Source: CAD feature listing. Evaluate the final solid. Frame: model axes, mm. A direction names the side the tool comes from. Coordinates: 2 decimals unless noted, no trailing zeros. Order: outer loops, then holes, each group sorted by start corner. A loop starts at its lowest first (then second) coordinate and runs counter-clockwise, first axis right, second up. Notation, with made-up numbers: (24.25, 28) - (73.25, 28) arc R31 ccw to (73.25, 62) - close; hole circle Ø3 at (66, 20.5). An arc over 180 degrees is marked (long way). One line per question, with ' | ' between items. Start each with the question number.
(1) Section A-A (y = 0). Return the cut outline in (x, z).
(2) Access query for faces 5 (the flat face through (25, 0, 0)), 6 (the cylindrical face through (15, 0, 0)). Directions: +Z, -Z, +X, -X, +Y, -Y. A direction counts if a zero-diameter tool reaches every point of the face in a straight line with its end or side. Return the directions, or none.
(3) Section B-B (x = 64). Return the cut outline in (y, z), then the cut area to 3 significant figures.
(4) Draft query along Z for faces 1 (the flat face through (100, 0, 0)), 2 (the flat face through (22, 0, -5)), 3 (the flat face through (20, 0, 0)), 4 (the cylindrical face through (46.835, 0.66, 14.985)). Return one class per face: +Z half, -Z half, draft (parallel to the pull), parting line (faces both ways), or undercut.
(5) Line query: line 1 along Z through (x, y) = (71, -0.5); line 2 along X through (y, z) = (1.5, -4.5); line 3 along X through (y, z) = (-11, -3.5). Output: solid intervals per line, ascending.
(6) Section C-C (x = 7.5). Return the cut outline in (y, z).
(7) Contact query for flat-ended pins moving along their axis: P1, Ø2, axis at x = 88.5, y = 11, coming from the -Z side; P2, Ø12, axis at x = 33, z = -9, coming from the +Y side; P3, Ø1, axis at x = 43.5, z = -2, coming from the -Y side. Output: stop coordinate, or through.
from build123d import *

# Parameters (mm, degrees)
BOX_W                = 5
BOX_H                = 10
BOX_DEPTH            = 48
BOX_ROLL_ANGLE       = 90
CYLINDER001_R        = 15
CYLINDER001_DEPTH    = 100
CYLINDER_R           = 15
CYLINDER_DEPTH       = 100
CYLINDER_PITCH_ANGLE = 90
FILLET_R             = 5


with BuildPart() as cubo:
    # Box → Box (new body)
    with BuildSketch(Plane.XY):
        with Locations((2.5, 5)):
            Rectangle(BOX_W, BOX_H)
    extrude(amount=BOX_DEPTH)


with BuildPart() as cubo_1:
    # Box roll: moved
    add(cubo.part.rotate(Axis((0, 0, 0), (1, 0, 0)), BOX_ROLL_ANGLE))


with BuildPart() as cubo_2:
    # Box placement: moved
    add(cubo_1.part.moved(Location((20, 27, -5))))


with BuildPart() as cilindro001:
    # Cylinder001 → Cylinder001 (new body)
    with BuildSketch(Plane.XY.offset(-44)):
        Circle(CYLINDER001_R)
    extrude(amount=CYLINDER001_DEPTH)


with BuildPart() as fillet_body:
    # Cylinder → Cylinder (new body)
    with BuildSketch(Plane.XY):
        Circle(CYLINDER_R)
    extrude(amount=CYLINDER_DEPTH)


with BuildPart() as fillet_body_1:
    # Cylinder pitch: moved
    add(fillet_body.part.rotate(Axis((0, 0, 0), (0, 1, 0)), CYLINDER_PITCH_ANGLE))


with BuildPart() as fillet_body_2:
    # Cylinder placement: moved
    add(fillet_body_1.part)

    # Cut: cut Cilindro001
    add(cilindro001.part, mode=Mode.SUBTRACT)

    # Cut001: cut Cubo
    add(cubo_2.part, mode=Mode.SUBTRACT)

    # Fillet
    fillet_edges = [fillet_body_2.edges().sort_by_distance(p)[0] for p in [
        (100, 0, 15),
    ]]
    fillet(fillet_edges, radius=FILLET_R)


solid = fillet_body_2.part
Response values:
1) outline: (15, -15) - (95, -15) arc R5 ccw to (100, -10) - (100, 10) arc R5 ccw to (95, 15) - (15, 15) - close; hole (20, -5) - (25, -5) - (25, 5) - (20, 5) - close
2) face 5: +Y, -Y | face 6: +Z, -Z, -X
3) outline: circle Ø30 at (0, 0) | area: 707 mm²
4) face 1: draft | face 2: undercut | face 3: undercut | face 4: parting line
5) line 1: z = -14.99 to 14.99 | line 2: x = 14.92 to 20, 25 to 100 | line 3: x = 10.2 to 20, 25 to 99.76
6) outline: (-12.99, -7.5) - (-12.99, 7.5) arc R15 ccw to start; (12.99, -7.5) arc R15 ccw to (12.99, 7.5) - close
7) P1: stops at z = -11.18 | P2: stops at y = 14.7 | P3: stops at y = -14.92
